```python
from build123d import *

# Parameters (mm, degrees)
F0_W     = 43
F0_H     = 65
F0_R     = 2.6
F1_DEPTH = 3.6
F2_R     = 5


with BuildPart() as f1:
    # F0 (on Front) → F1 (new body)
    with BuildSketch(Plane.XZ):
        with Locations((0, -5.247028)):
            Rectangle(F0_W, F0_H)
        with Locations((-13.5, -28.747028)):
            Circle(F0_R, mode=Mode.SUBTRACT)
        with BuildLine():
            ThreePointArc((-17.25, -9.247028), (-15.5, -7.497028), (-13.75, -9.247028))
            Line((-13.75, -9.247028), (-13.75, -14.247028))
            ThreePointArc((-13.75, -14.247028), (-15.5, -15.997028), (-17.25, -14.247028))
            Line((-17.25, -14.247028), (-17.25, -9.247028))
        make_face(mode=Mode.SUBTRACT)
        with Locations((13.5, -28.747028)):
            Circle(F0_R, mode=Mode.SUBTRACT)
        with BuildLine():
            ThreePointArc((13.75, -9.247028), (15.5, -7.497028), (17.25, -9.247028))
            Line((17.25, -9.247028), (17.25, -14.247028))
            ThreePointArc((17.25, -14.247028), (15.5, -15.997028), (13.75, -14.247028))
            Line((13.75, -14.247028), (13.75, -9.247028))
        make_face(mode=Mode.SUBTRACT)
        with BuildLine():
            ThreePointArc((-17.25, 21.752972), (-15.5, 23.502972), (-13.75, 21.752972))
            Line((-13.75, 21.752972), (-13.75, 16.752972))
            ThreePointArc((-13.75, 16.752972), (-15.5, 15.002972), (-17.25, 16.752972))
            Line((-17.25, 16.752972), (-17.25, 21.752972))
        make_face(mode=Mode.SUBTRACT)
        with BuildLine():
            ThreePointArc((11.1, 1.252972), (0, -9.847028), (-11.1, 1.252972))
            Line((-11.1, 1.252972), (-11.1, 6.252972))
            ThreePointArc((-11.1, 6.252972), (0, 17.352972), (11.1, 6.252972))
            Line((11.1, 6.252972), (11.1, 1.252972))
        make_face(mode=Mode.SUBTRACT)
        with BuildLine():
            ThreePointArc((13.75, 21.752972), (15.5, 23.502972), (17.25, 21.752972))
            Line((17.25, 21.752972), (17.25, 16.752972))
            ThreePointArc((17.25, 16.752972), (15.5, 15.002972), (13.75, 16.752972))
            Line((13.75, 16.752972), (13.75, 21.752972))
        make_face(mode=Mode.SUBTRACT)
    extrude(amount=F1_DEPTH)

    # F2
    f2_edges = [f1.edges().sort_by_distance(p)[0] for p in [
        (-21.5, -1.8, 27.252972),
        (21.5, -1.8, 27.252972),
    ]]
    fillet(f2_edges, radius=F2_R)


solid = f1.part
```
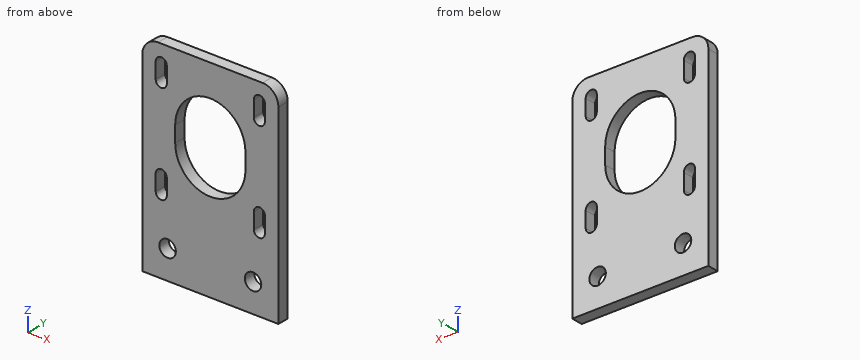
The listing builds one solid part. Answer for the finished solid, in the listing's coordinates (mm). Give positions to 0.01 mm unless a question says otherwise; leave off trailing zeros. Loops run counter-clockwise (first coordinate to the right, second up) from the corner with the lowest first, then second, coordinate; pieces in that order, holes last. Notation, with made-up numbers: M 20.5,-37.75 L 55.5,-37.75 A7 cw 55.5,-24.75 Z; hole C 6,-22 d4. An arc over 180 degrees is marked long. One line per item, written item: value.
Q1. A cutting plane is placed at A-A on y = -0.6. Determine the outline of the cut face in (x, z).
Working result:
outline: M -21.5,-37.75 L 21.5,-37.75 L 21.5,22.25 A5 ccw 16.5,27.25 L -16.5,27.25 A5 ccw -21.5,22.25 Z; hole M -17.25,-14.25 A1.75 ccw -13.75,-14.25 L -13.75,-9.25 A1.75 ccw -17.25,-9.25 Z; hole M -17.25,16.75 A1.75 ccw -13.75,16.75 L -13.75,21.75 A1.75 ccw -17.25,21.75 Z; hole C -13.5,-28.75 d5.2; hole M -11.1,1.25 A11.1 ccw 11.1,1.25 L 11.1,6.25 A11.1 ccw -11.1,6.25 Z; hole C 13.5,-28.75 d5.2; hole M 13.75,-14.25 A1.75 ccw 17.25,-14.25 L 17.25,-9.25 A1.75 ccw 13.75,-9.25 Z; hole M 13.75,16.75 A1.75 ccw 17.25,16.75 L 17.25,21.75 A1.75 ccw 13.75,21.75 Z
Q2. A cutting plane is placed at B-B on x = 13. Determine the outline of the cut face in (y, z).
Working result:
outline: M -3.6,-37.75 L 0,-37.75 L 0,-31.3 L -3.6,-31.3 Z; M -3.6,-26.2 L 0,-26.2 L 0,27.25 L -3.6,27.25 Z
Q3. A flat-ended cylindrical pin translates along its axis: P1, Ø4.5, axis at x = 13.5, z = -28.75, coming from the -Y side. Find the tip coordinate at first contact, or state that the pin passes through.
Working result:
P1: passes through
Q4. Find the intervals of material crossed by line 1 (X direction, y = -1.75, z = -10); line 2 (X direction, y = -1.35, z = -30.5); line 3 (Z direction, x = 13.5, y = -2.7), in increasing order. Write a range as from..to.
Working result:
line 1: x = -21.5..-17.25, -13.75..13.75, 17.25..21.5
line 2: x = -21.5..-15.42, -11.58..11.58, 15.42..21.5
line 3: z = -37.75..-31.35, -26.15..27.25
